The listing builds one solid part. Answer for the finished solid, in the listing's coordinates (mm). A direction names the side the tool comes from. Round coordinates to 2 decimals unless told otherwise and drop trailing zeros. Write each loop counter-clockwise with the first axis right and the second up, starting at its lowest first coordinate (ties: lowest second). Pieces come first, ordered by that corner, then holes. Notation, with made-up numbers: (57.5, 24.25) - (94.5, 24.25) arc R6 ccw to (94.5, 30.25) - close; hole circle Ø7 at (30.25, 58). An arc over 180 degrees is marked (long way). Return JSON: item names as keys, results as strings. Group by question number.
(1) Section A-A, the plane x = 0 is taken. Write down the section's boundary in (y, z).
(2) Determine the mould class of faces 1 (the cylindrical face through (-7.99, 0.07, 6.15)), 2 (the cylindrical face through (1.93, -0.8, 10.44)), 3 (the flat face through (-3, 1, 5)), 4 (the flat face through (-3, 4, 11)) for opening direction Y: +Y half, -Y half, draft (parallel to the pull), parting line (faces both ways), or undercut.
(3) Section B-B, the plane x = -4.5 is taken. Write down the section's boundary in (y, z), then the cut area to 3 significant figures.
(4) Section D-D, the plane z = 2.75 is taken. Write down the section's boundary in (x, y) (3 decimals), then the cut area to 3 significant figures.
(5) Each of these flat-tipped pins is pushed along its axis until it touches: pin 1 (4 mm diameter, centred on y = 0, z = 3.15, fed in from +X); pin 2 (2 mm diameter, centred on y = -1.5, z = 3, fed in from +X); pin 3 (1.5 mm diameter, centred on x = 3, z = 3.5, fed in from -Y). Where does it stop, or does it pass through?
(6) Which of the six approach directions +Z, -Z, +X, -X, +Y, -Y give full straight-line access (tool end or side, diameter ignored) to faces 5 (the flat face through (0.5, -1, 5)), 6 (the cylindrical face through (-4.931, -1.641, 10.646)), 7 (the flat face through (-7, -1, 5))?
(7) Find the intervals of material crossed by line 1 along Y through (x, z) = (-1.5, 13.75); line 2 along Y through (x, z) = (0, 12.25); line 3 along X through (y, z) = (-1, 4.5), in increasing order. Write a range as [from, to].
(8) Section C-C, the plane y = -0.75 is taken. Write down the section's boundary in (x, z), then the cut area to 3 significant figures.
```python
from build123d import *

# Parameters (mm, degrees)
SCHIZZO1_R                           = 2.09
ESTRUSIONE_ESTRUSIONE1_DEPTH         = 15
SCHIZZO5_W                           = 3.5
SCHIZZO5_H                           = 7.5
TAGLIO_ESTRUSIONE4_DEPTH             = 9
ESTRUSIONE_ESTRUSIONE2_REACH         = 7.492
SCHIZZO6_W                           = 6
SCHIZZO6_H                           = 8
SCHIZZO7_R                           = 1.45
TAGLIO_ESTRUSIONE5_DEPTH             = 9.992075583
TAGLIO_ESTRUSIONE5_DEPTH_BACK        = 7.000142198
SCHIZZO7_4_R                         = 1.85
TAGLIO_ESTRUSIONE6_DEPTH             = 7.000142323
TAGLIO_ESTRUSIONE6_DIRECTION_2_REACH = 10.992
RACCORDO1_R                          = 0.7
RACCORDO2_R                          = 0.7
TAGLIO_ESTRUSIONE7_DEPTH             = 8.179825842
TAGLIO_ESTRUSIONE7_DEPTH_BACK        = 7.000142323
TAGLIO_ESTRUSIONE9_START             = -4
SCHIZZO9_R                           = 3
TAGLIO_ESTRUSIONE9_DEPTH             = 3.000142323


with BuildPart() as part:
    # Schizzo1 → Estrusione-Estrusione1 (new body)
    with BuildSketch(Plane.XY):
        with BuildLine():
            Line((5.992217781, -4), (-8.491933385, -4))
            ThreePointArc((-8.491933385, -4), (-9, 0), (-8.491933385, 4))
            Line((-8.491933385, 4), (5.992217781, 4))
            ThreePointArc((5.992217781, 4), (2.875, 0), (5.992217781, -4))
        make_face()
        Circle(SCHIZZO1_R, mode=Mode.SUBTRACT)
    extrude(amount=ESTRUSIONE_ESTRUSIONE1_DEPTH)

    # Schizzo5 → Taglio-Estrusione4 (cut, through all)
    with BuildSketch(Plane.XZ.offset(4)):
        with Locations((-1.249857802, 3.75)):
            Rectangle(SCHIZZO5_W, SCHIZZO5_H)
    extrude(amount=-TAGLIO_ESTRUSIONE4_DEPTH, mode=Mode.SUBTRACT)

    # Schizzo6 → Estrusione-Estrusione2 (add, up to next)
    with BuildSketch(Plane.ZY.offset(-0.500142198), mode=Mode.PRIVATE) as estrusione_estrusione2_sk1:
        with Locations((3, 0)):
            Rectangle(SCHIZZO6_W, SCHIZZO6_H)
    estrusione_estrusione2_tool1 = extrude(estrusione_estrusione2_sk1.sketch, amount=-ESTRUSIONE_ESTRUSIONE2_REACH, mode=Mode.PRIVATE) - part.part
    add(estrusione_estrusione2_tool1.solids().sort_by_distance((0.500142, 0, 3))[0])

    # Schizzo7 → Taglio-Estrusione5 (cut, two sides)
    with BuildSketch(Plane(origin=(-2.999857802, 0, 0), x_dir=(0, 0, -1), z_dir=(1, 0, 0))) as taglio_estrusione5_sk:
        with Locations((-3.15, 0)):
            Circle(SCHIZZO7_R)
    extrude(amount=TAGLIO_ESTRUSIONE5_DEPTH, mode=Mode.SUBTRACT)
    extrude(taglio_estrusione5_sk.sketch, amount=-TAGLIO_ESTRUSIONE5_DEPTH_BACK, mode=Mode.SUBTRACT)

    # Schizzo7<4> → Taglio-Estrusione6 (cut)
    with BuildSketch(Plane(origin=(-2.999857802, 0, 0), x_dir=(0, 0, -1), z_dir=(1, 0, 0))):
        with Locations((-11.5, 0)):
            Circle(SCHIZZO7_4_R)
    extrude(amount=-TAGLIO_ESTRUSIONE6_DEPTH, mode=Mode.SUBTRACT)

    # Schizzo7<4> → Taglio-Estrusione6 direction 2 (cut, up to next)
    with BuildSketch(Plane(origin=(-2.999857802, 0, 0), x_dir=(0, 0, -1), z_dir=(1, 0, 0)), mode=Mode.PRIVATE) as taglio_estrusione6_direction_2_sk1:
        with Locations((-11.5, 0)):
            Circle(SCHIZZO7_4_R)
    taglio_estrusione6_direction_2_tool1 = extrude(taglio_estrusione6_direction_2_sk1.sketch, amount=TAGLIO_ESTRUSIONE6_DIRECTION_2_REACH, mode=Mode.PRIVATE) & part.part
    add(taglio_estrusione6_direction_2_tool1.solids().sort_by_distance((-2.999858, 0, 11.5))[0], mode=Mode.SUBTRACT)

    # Raccordo1
    raccordo1_edges = [part.edges().sort_by_distance(p)[0] for p in [
        (5.992217781, 4, 7.5),
    ]]
    fillet(raccordo1_edges, radius=RACCORDO1_R)

    # Raccordo2
    raccordo2_edges = [part.edges().sort_by_distance(p)[0] for p in [
        (5.992217781, -4, 7.5),
    ]]
    fillet(raccordo2_edges, radius=RACCORDO2_R)

    # Schizzo8 → Taglio-Estrusione7 (cut, two sides)
    with BuildSketch(Plane(origin=(-2.999857802, 0, 0), x_dir=(0, 0, -1), z_dir=(1, 0, 0))) as taglio_estrusione7_sk:
        with BuildLine():
            Line((-3.15, -4), (0, -4))
            Line((0, -4), (0, 4))
            Line((0, 4), (-3.15, 4))
            Line((-3.15, 4), (-7.5, 4))
            Line((-7.5, 4), (-3.15, 3))
            ThreePointArc((-3.15, 3), (-0.15, 0), (-3.15, -3))
            Line((-3.15, -3), (-7.5, -4))
            Line((-7.5, -4), (-3.15, -4))
        make_face()
    extrude(amount=TAGLIO_ESTRUSIONE7_DEPTH, mode=Mode.SUBTRACT)
    extrude(taglio_estrusione7_sk.sketch, amount=-TAGLIO_ESTRUSIONE7_DEPTH_BACK, mode=Mode.SUBTRACT)

    # Schizzo9 → Taglio-Estrusione9 (cut, through all)
    with BuildSketch(Plane(origin=(-2.999857802, 0, 0), x_dir=(0, 0, -1), z_dir=(1, 0, 0)).offset(TAGLIO_ESTRUSIONE9_START)):
        with Locations((-3.15, 0)):
            Circle(SCHIZZO9_R)
    extrude(amount=-TAGLIO_ESTRUSIONE9_DEPTH, mode=Mode.SUBTRACT)


solid = part.part
```
Working result:
{
 "1": {"outline": "(-4, 7.5) - (-2.09, 7.5) - (-2.09, 15) - (-4, 15) - close; (2.09, 7.5) - (4, 7.5) - (4, 15) - (2.09, 15) - close"},
 "2": {"face 1": "undercut", "face 2": "undercut", "face 3": "draft", "face 4": "+Y half"},
 "3": {"outline": "(-4, 7.5) - (-3, 3.15) arc R3 ccw to (3, 3.15) - (4, 7.5) - (4, 15) - (-4, 15) - close; hole circle Ø3.7 at (0, 11.5); hole circle Ø2.9 at (0, 3.15)", "area": "87.2 mm^2"},
 "4": {"outline": "(-7, -2.973) - (-3, -2.973) - (-3, -1.394) - (-7, -1.394) - close; (-7, 1.394) - (-3, 1.394) - (-3, 2.973) - (-7, 2.973) - close; (0.5, -2.973) - (4.099, -2.973) arc R0.7 ccw to (3.991, -2.821) arc R4.125 cw to (3.118, -1.394) - (0.5, -1.394) - close; (0.5, 1.394) - (3.118, 1.394) arc R4.125 cw to (3.991, 2.821) arc R0.7 ccw to (4.099, 2.973) - (0.5, 2.973) - close", "area": "22.2 mm^2"},
 "5": {"pin 1": "stops at x = 3.39", "pin 2": "stops at x = 3.72", "pin 3": "stops at y = -3.25"},
 "6": {"face 5": "-Z, +Y, -Y", "face 6": "-X", "face 7": "-Z, -X"},
 "7": {"line 1": "y = [-4, -1.46], [1.46, 4]", "line 2": "y = [-4, -2.09], [2.09, 4]", "line 3": "x = [-7, -3], [0.5, 3]"},
 "8": {"outline": "(-8.98, 6.05) - (-7, 6.05) - (-7, 4.39) - (-3, 4.39) - (-3, 7.5) - (-1.95, 7.5) - (-1.95, 9.81) - (-8.98, 9.81) - close; (-8.98, 13.19) - (-1.95, 13.19) - (-1.95, 15) - (-8.98, 15) - close; (-7, 0.25) - (-3, 0.25) - (-3, 1.91) - (-7, 1.91) - close; (0.5, 0.25) - (2.94, 0.25) - (2.94, 1.91) - (0.5, 1.91) - close; (0.5, 4.39) - (2.94, 4.39) - (2.94, 15) - (1.95, 15) - (1.95, 6) - (0.5, 6) - close", "area": "67.8 mm^2"}
}
